Autodesk Fusion 360 part; units mm, degrees
sketch "Sketch1" plane through (0, 0, 0) normal (0, 0, 1) x (1, 0, 0)
  circle A0 centre (0, 0) radius 42.75
  circle A1 centre (0, 0) radius 39.5
  line L0 (0, 0) -> (0, -100) construction
  line L1 (100, -105) -> (-100, -105)
  line L2 (-100, -105) -> (-100, -95)
  line L3 (100, -95) -> (100, -105)
  line L4 (100, -105) -> (-100, -95) construction
  line L5 (-100, -105) -> (100, -95) construction
  circle A2 centre (0, 0) radius 52.5
  line L6 (-52.5, 0) -> (-52.5, -57.5)
  line L7 (52.5, 0) -> (52.5, -57.5)
  line L8 (-100, -95) -> (-90, -95)
  line L9 (90, -95) -> (100, -95)
  arc A3 (-90, -95) -> (-52.5, -57.5) centre (-90, -57.5) ccw
  arc A4 (52.5, -57.5) -> (90, -95) centre (90, -57.5) ccw
  point P0 (0, -100)
  dimension "d1" = 85.5
  dimension "d5" = 79
  dimension "d7" = 100
  dimension "d8" = 200
  dimension "d9" = 10
  dimension "d10" = 105
  dimension "d11" = 37.5
  dimension "d12" = 10
  dimension "d13" = 37.5
extrude "Extrude1" add sketch "Sketch1" along normal blind 12 contours L1 L2 L3 A2 L6 L7 L8 L9 A3 A4 | A2
extrude "Extrude2" add sketch "Sketch1" along normal blind 2 contours A0
hole "Hole1" at (-95, -95, 6) direction (0, -1, 0) diameter 3 depth 10 tip angle 118
hole "Hole2" at (95.5037, -95, 6.5484) direction (0, -1, 0) diameter 3 depth 10 tip angle 118
equation "d1 = BearingDia + Tollerance"
equation "BearingDia = 85 mm"
equation "BearingOffset = 79 mm"
equation "Tollerance = 0.5 mm"
equation "d5 = BearingOffset"
equation "AxleHeight = 105 mm"
equation "d7 = AxleHeight - 5 mm"
equation "d10 = BearingDia + 20 mm"
Can you work these out from the model? Positions are in its coordinate system, mm. A direction names the side the tool comes from. Give positions to 0.01 mm unless a question says otherwise; leave off trailing zeros. Order: outer loops, then holes, each group sorted by start corner. A loop starts at its lowest first (then second) coordinate and runs counter-clockwise, first axis right, second up. Notation, with made-up numbers: M 35.25,58 L 61.25,58 A26 ccw 61.25,96 Z; hole C 17.5,-26.75 d4. An arc over 180 degrees is marked long. One line per item, written item: value.
Item 1: If we section it at D-D on y = -90.5: Write out the boundary of the cut face in (x, z), and give its area (3 significant figures).
Verdict:
outline: M -72.19,0 L 72.19,0 L 72.19,12 L -72.19,12 Z
area: 1,730 mm2
Item 2: If we mould it in two halves opening along X, with no side actions, what happens to faces 5 (the face through (-1.154, 52.487, 5.916)), 6 (the face through (40.776, -12.841, 6.93)), 7 (the face through (-1, -43, 0)), 8 (the face through (-29.11, -26.7, 0.99))? For each: pulls with the +X half, pulls with the -X half, needs draft (parallel to the pull), parting line crosses it, or undercut.
Verdict:
face 5: parting line crosses it
face 6: undercut
face 7: needs draft
face 8: undercut
Item 3: If we section it at A-A on x = 0: Write out the boundary of the cut face in (y, z), and give its area (3 significant figures).
Verdict:
outline: M -105,0 L -39.5,0 L -39.5,2 L -42.75,2 L -42.75,12 L -105,12 Z; M 39.5,0 L 52.5,0 L 52.5,12 L 42.75,12 L 42.75,2 L 39.5,2 Z
area: 877 mm2
Item 4: For pin 1 (4 mm diameter, centred on x = 63.5, z = 9.5, fed in from +Y); pin 2 (4 mm diameter, centred on y = 17.5, z = 5.5, fed in from +X); pin 3 (1.8 mm diameter, centred on x = -95, z = 6, fed in from +Y); pin 4 (5 mm diameter, centred on x = 34, y = -20, fed in from +Z), each with a flat end and sliding along its axis, tell me the tip position at first contact or that it passes through.
Verdict:
pin 1: y = -81.87
pin 2: x = 50.16
pin 3: through
pin 4: z = 2
Item 5: If we section it at C-C on x = -62: Write out the boundary of the cut face in (y, z), and give its area (3 significant figures).
Verdict:
outline: M -105,0 L -82.44,0 L -82.44,12 L -105,12 Z
area: 271 mm2
Item 6: If we section it at B-B on y = -28.5: Write out the boundary of the cut face in (x, z).
Verdict:
outline: M -52.5,0 L -27.35,0 L -27.35,2 L -31.86,2 L -31.86,12 L -52.5,12 Z; M 27.35,0 L 52.5,0 L 52.5,12 L 31.86,12 L 31.86,2 L 27.35,2 Z
Item 7: For faces 1 (the face through (38, -12, 2)), 2 (the face through (93.8, -95, 5.9)), 3 (the face through (-96.2, -95, 4.6)), 4 (the face through (-1, -60, 12)), which set-ups out of +Z, -Z, +X, -X, +Y, -Y let a thin tool reach every point of the face, with its end or its side?
Verdict:
face 1: +Z
face 2: +Z, -Z, +X, +Y
face 3: +Z, -Z, -X, +Y
face 4: +Z, +X, -X, +Y, -Y
Item 8: Please list where these lines run through material, in increasing order: line 1 (Y direction, x = 0, z = 1.5); line 2 (X direction, y = -101.5, z = 6); line 3 (Y direction, x = 88.5, z = 6.25).
Verdict:
line 1: -105 to -39.5, 39.5 to 52.5
line 2: -100 to -96.5, -93.5 to 94.11, 96.9 to 100
line 3: -105 to -94.97
